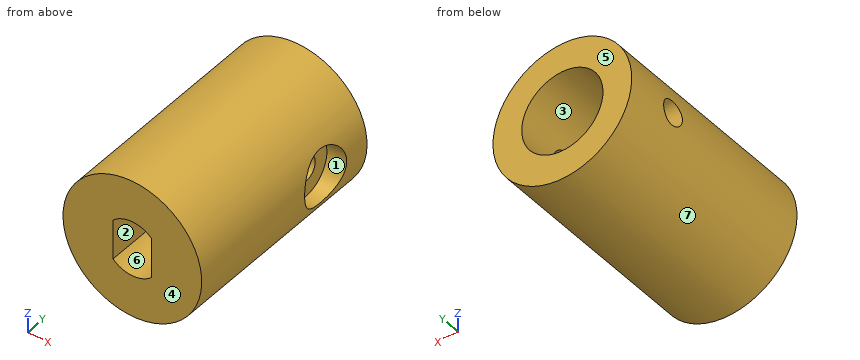
```python
from build123d import *

# Parameters (mm, degrees)
SKETCH1_R                               = 7
BOSS_EXTRUDE1_DEPTH                     = 22
SKETCH2_R                               = 4.1
CUT_EXTRUDE1_DEPTH                      = 14
CUT_EXTRUDE2_DEPTH                      = 8
CBORE_FOR_M5_HEX_HEAD_BOLT1_D           = 2.5
CBORE_FOR_M5_HEX_HEAD_BOLT1_CBORE_D     = 5.6
CBORE_FOR_M5_HEX_HEAD_BOLT1_CBORE_DEPTH = 2


with BuildPart() as part:
    # Sketch1 → Boss-Extrude1 (new body)
    with BuildSketch(Plane(origin=(0, 0, 0), x_dir=(1, 0, 0), z_dir=(0, 1, 0))):
        with Locations(Location((0, 0, 0), (0, 0, 270))):
            Circle(SKETCH1_R)
    extrude(amount=BOSS_EXTRUDE1_DEPTH)

    # Sketch2 → Cut-Extrude1 (cut)
    with BuildSketch(Plane(origin=(0, 22, 0), x_dir=(1, 0, 0), z_dir=(0, 1, 0))):
        with Locations(Location((0, 0, 0), (0, 0, 270))):
            Circle(SKETCH2_R)
    extrude(amount=-CUT_EXTRUDE1_DEPTH, mode=Mode.SUBTRACT)

    # Sketch3 → Cut-Extrude2 (cut)
    with BuildSketch(Plane.XZ):
        with BuildLine():
            Line((-1.95, 2.00935313), (-1.95, -2.00935313))
            ThreePointArc((-1.95, -2.00935313), (0, -2.8), (1.95, -2.00935313))
            Line((1.95, -2.00935313), (1.95, 2.00935313))
            ThreePointArc((1.95, 2.00935313), (0, 2.8), (-1.95, 2.00935313))
        make_face()
    extrude(amount=-CUT_EXTRUDE2_DEPTH, mode=Mode.SUBTRACT)

    # CBORE for M5 Hex Head Bolt1 (through all)
    with Locations(Plane(origin=(7, 16.5, 0), x_dir=(0, 0, 1), z_dir=(1, 0, 0))):
        with Locations((0, 0)):
            CounterBoreHole(CBORE_FOR_M5_HEX_HEAD_BOLT1_D / 2, CBORE_FOR_M5_HEX_HEAD_BOLT1_CBORE_D / 2, CBORE_FOR_M5_HEX_HEAD_BOLT1_CBORE_DEPTH)


solid = part.part
```
Input: part model. Units: mm. Frame: model coordinates. Face numbers are marked on the shaded views. A direction names the side the tool comes from. Give positions to 0.01 mm unless a question says otherwise; leave off trailing zeros. Order: outer loops, then holes, each group sorted by start corner. A loop starts at its lowest first (then second) coordinate and runs counter-clockwise, first axis right, second up. Notation, with made-up numbers: (74, 10.25) - (104, 10.25) arc R16 cw to (104, 23.25) - close; hole circle Ø4 at (43, 9.25). An arc over 180 degrees is marked (long way). One line per item, written item: value.
1. Pin query (flat end, axial travel): pin 1 Ø1.5 at (y, z) = (16.5, 0) entering from +X; pin 2 Ø6 at (x, y) = (-3.5, 16.5) entering from -Z; pin 3 Ø1.5 at (x, y) = (-3.5, 15) entering from -Z; pin 4 Ø4 at (x, z) = (0, -1.5) entering from +Y. Return the tip coordinate at first contact, or that it passes through.
Determined:
pin 1: through
pin 2: z = -6.98
pin 3: z = -6.44
pin 4: y = 8
2. Cut plane D-D, the plane y = 7. Output: boundary loops of the cut face in (x, z).
Determined:
outline: circle Ø14 at (0, 0); hole (-1.95, -2.01) arc R2.8 ccw to (1.95, -2.01) - (1.95, 2.01) arc R2.8 ccw to (-1.95, 2.01) - close
3. Draft query along X for the marked faces 5, 6 and 7. Return one class per face: released by +X, released by -X, zero draft, split by the parting line, or undercut.
Determined:
face 5: zero draft
face 6: undercut
face 7: split by the parting line
4. Cut plane A-A, the plane z = 0. Output: boundary loops of the cut face in (x, y), and give its area (3 significant figures).
Determined:
outline: (-7, 0) - (-1.95, 0) - (-1.95, 8) - (-4.1, 8) - (-4.1, 15.25) - (-7, 15.25) - close; (-7, 17.75) - (-4.1, 17.75) - (-4.1, 22) - (-7, 22) - close; (1.95, 0) - (7, 0) - (7, 13.7) - (5, 13.7) - (5, 15.25) - (4.1, 15.25) - (4.1, 8) - (1.95, 8) - close; (4.1, 17.75) - (5, 17.75) - (5, 19.3) - (7, 19.3) - (7, 22) - (4.1, 22) - close
area: 141 mm2
5. Line query: probe 1 along Y at (x, z) = (-4.75, 0); probe 2 along Y at (x, z) = (-2.25, 3.25); probe 3 along X at (y, z) = (17.25, -2.75). Output: solid intervals per line, ascending.
Determined:
probe 1: 0 to 15.25, 17.75 to 22
probe 2: 0 to 8
probe 3: -6.44 to -3.04, 3.04 to 6.44
6. Reachability of the marked faces 1, 2, 3 and 4 from +Z, -Z, +X, -X, +Y, -Y: full face, straight path, thin tool, end or side. Return the list, or none.
Determined:
face 1: +X
face 2: +Y, -Y
face 3: +Y
face 4: +Z, -Z, +X, -X, -Y
7. Cut plane C-C, the plane z = 1.75. Output: boundary loops of the cut face in (x, y).
Determined:
outline: (-6.78, 0) - (-1.95, 0) - (-1.95, 8) - (-3.71, 8) - (-3.71, 22) - (-6.78, 22) - close; (1.95, 0) - (6.78, 0) - (6.78, 14.31) - (5, 14.31) - (5, 18.69) - (6.78, 18.69) - (6.78, 22) - (3.71, 22) - (3.71, 8) - (1.95, 8) - close
8. Cut plane B-B, the plane y = 16.5. Output: boundary loops of the cut face in (x, z).
Determined:
outline: (-6.89, -1.25) arc R7 ccw to (6.42, -2.8) - (5, -2.8) - (5, -1.25) - (3.9, -1.25) arc R4.1 cw to (-3.9, -1.25) - close; (-6.89, 1.25) - (-3.9, 1.25) arc R4.1 cw to (3.9, 1.25) - (5, 1.25) - (5, 2.8) - (6.42, 2.8) arc R7 ccw to start
